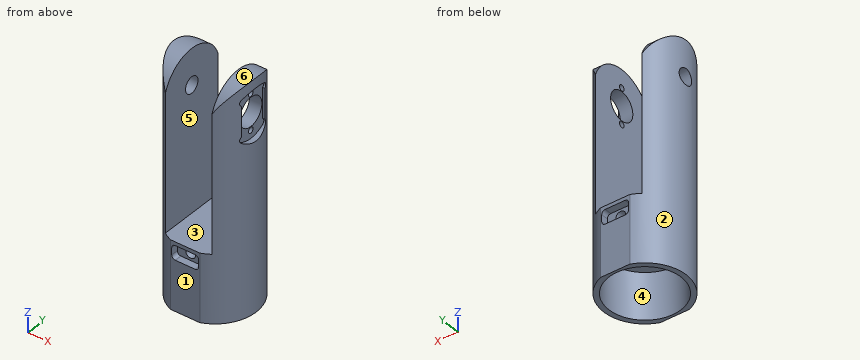
from build123d import *

# Parameters (mm, degrees)
F1_DEPTH  = 128
F3_W      = 26
F3_H      = 46
F4_DEPTH  = 90
F6_DEPTH  = 46.001
F8_DEPTH  = 3
F10_D     = 3.3
F10_DEPTH = 20
F10_TIP   = 0.9914200214
F11_R     = 8
F12_DEPTH = 25
F13_R     = 4.5
F14_DEPTH = 10.0010001
F15_R     = 20.15
F16_DEPTH = 26
F18_DEPTH = 4
F20_D     = 5.5
F20_DEPTH = 10
F20_TIP   = 1.6523667023
F22_DEPTH = 4
F24_D     = 5.5
F24_DEPTH = 10
F24_TIP   = 1.6523667023


with BuildPart() as f1:
    # F0 (on Top) → F1 (new body)
    with BuildSketch(Plane.XY):
        with BuildLine():
            Line((8.1700673192, 21.5), (-8.1700673192, 21.5))
            ThreePointArc((-8.1700673192, 21.5), (-23, 0), (-8.1700673192, -21.5))
            Line((-8.1700673192, -21.5), (8.1700673192, -21.5))
            ThreePointArc((8.1700673192, -21.5), (23, 0), (8.1700673192, 21.5))
        make_face()
    extrude(amount=F1_DEPTH)

    # F3 (on face) → F4 (cut)
    with BuildSketch(Plane.XY.offset(128)):
        Rectangle(F3_W, F3_H)
    extrude(amount=-F4_DEPTH, mode=Mode.SUBTRACT)

    # F5 (on offset) → F6 (cut, through all)
    with BuildSketch(Plane.YZ.offset(23)):
        with BuildLine():
            ThreePointArc((-19.9933908829, 108.5141215848), (-0.0190112138, 127.9999909643), (19.9923773451, 108.5521305014))
            Line((19.9923773451, 108.5521305014), (24.1833440959, 131.3719953258))
            Line((24.1833440959, 131.3719953258), (-19.9933908829, 131.3719953258))
            Line((-19.9933908829, 131.3719953258), (-19.9933908829, 108.5141215848))
        make_face()
    extrude(amount=-F6_DEPTH, mode=Mode.SUBTRACT)

    # F7 (on offset) → F8 (cut)
    with BuildSketch(Plane.YZ.offset(23)):
        with BuildLine():
            ThreePointArc((-8.55, 99.5196213389), (-9.3706896552, 97.9043111178), (-8.55, 96.2890008966))
            ThreePointArc((-8.55, 96.2890008966), (0, 93.5), (8.55, 96.2890008966))
            ThreePointArc((8.55, 96.2890008966), (9.3706896552, 97.9043111178), (8.55, 99.5196213389))
            Line((8.55, 99.5196213389), (8.55, 116.4803786611))
            ThreePointArc((8.55, 116.4803786611), (9.3706896552, 118.0956888822), (8.55, 119.7109991034))
            ThreePointArc((8.55, 119.7109991034), (0, 122.5), (-8.55, 119.7109991034))
            ThreePointArc((-8.55, 119.7109991034), (-9.3706896552, 118.0956888822), (-8.55, 116.4803786611))
            Line((-8.55, 116.4803786611), (-8.55, 99.5196213389))
        make_face()
    extrude(amount=-F8_DEPTH, mode=Mode.SUBTRACT)

    # F10
    with Locations(Plane.YZ.offset(20)):
        with Locations((0, 118), (0, 98)):
            Hole(F10_D / 2, depth=F10_DEPTH)
            with Locations((0, 0, -(F10_DEPTH + F10_TIP / 2))):  # 118° drill point
                Cone(0, F10_D / 2, F10_TIP, mode=Mode.SUBTRACT)

    # F11 (on face) → F12 (cut)
    with BuildSketch(Plane.YZ.offset(20)):
        with Locations((0, 108)):
            Circle(F11_R)
    extrude(amount=-F12_DEPTH, mode=Mode.SUBTRACT)

    # F13 (on face) → F14 (cut, through all)
    with BuildSketch(Plane.YZ.offset(-13)):
        with Locations((0, 108)):
            Circle(F13_R)
    extrude(amount=-F14_DEPTH, mode=Mode.SUBTRACT)

    # F15 (on face) → F16 (cut)
    with BuildSketch(Plane(origin=(0, 0, 0), x_dir=(1, 0, 0), z_dir=(0, 0, -1))):
        Circle(F15_R)
    extrude(amount=-F16_DEPTH, mode=Mode.SUBTRACT)

    # F17 (on face) → F18 (cut)
    with BuildSketch(Plane.XZ.offset(21.5)):
        with BuildLine():
            Line((5.5, 36), (-5.5, 36))
            ThreePointArc((-5.5, 36), (-6.9142135624, 35.4142135624), (-7.5, 34))
            Line((-7.5, 34), (-7.5, 30))
            ThreePointArc((-7.5, 30), (-6.9142135624, 28.5857864376), (-5.5, 28))
            Line((-5.5, 28), (5.5, 28))
            ThreePointArc((5.5, 28), (6.9142135624, 28.5857864376), (7.5, 30))
            Line((7.5, 30), (7.5, 34))
            ThreePointArc((7.5, 34), (6.9142135624, 35.4142135624), (5.5, 36))
        make_face()
    extrude(amount=-F18_DEPTH, mode=Mode.SUBTRACT)

    # F20
    with Locations(Plane.XZ.offset(17.5)):
        with Locations((0, 32)):
            Hole(F20_D / 2, depth=F20_DEPTH)
            with Locations((0, 0, -(F20_DEPTH + F20_TIP / 2))):  # 118° drill point
                Cone(0, F20_D / 2, F20_TIP, mode=Mode.SUBTRACT)

    # F21 (on face) → F22 (cut)
    with BuildSketch(Plane(origin=(0, 21.5, 0), x_dir=(-1, 0, 0), z_dir=(0, 1, 0))):
        with BuildLine():
            Line((5.5, 36), (-5.5, 36))
            ThreePointArc((-5.5, 36), (-6.9142135624, 35.4142135624), (-7.5, 34))
            Line((-7.5, 34), (-7.5, 30))
            ThreePointArc((-7.5, 30), (-6.9142135624, 28.5857864376), (-5.5, 28))
            Line((-5.5, 28), (5.5, 28))
            ThreePointArc((5.5, 28), (6.9142135624, 28.5857864376), (7.5, 30))
            Line((7.5, 30), (7.5, 34))
            ThreePointArc((7.5, 34), (6.9142135624, 35.4142135624), (5.5, 36))
        make_face()
    extrude(amount=-F22_DEPTH, mode=Mode.SUBTRACT)

    # F24
    with Locations(Plane(origin=(0, 17.5, 0), x_dir=(-1, 0, 0), z_dir=(0, 1, 0))):
        with Locations((0, 32)):
            Hole(F24_D / 2, depth=F24_DEPTH)
            with Locations((0, 0, -(F24_DEPTH + F24_TIP / 2))):  # 118° drill point
                Cone(0, F24_D / 2, F24_TIP, mode=Mode.SUBTRACT)


solid = f1.part
Input: part model. Units: mm. Frame: model coordinates. Face numbers are marked on the shaded views. A direction names the side the tool comes from. Give positions to 0.01 mm unless a question says otherwise; leave off trailing zeros. Order: outer loops, then holes, each group sorted by start corner. A loop starts at its lowest first (then second) coordinate and runs counter-clockwise, first axis right, second up. Notation, with made-up numbers: M -25,53 L 32,53 A35 ccw 32,87 Z; hole C -14,2.25 d7. An arc over 180 degrees is marked long. Answer as a JSON object with one key per item and string values.
1. Cut plane B-B, the plane z = 12.5. Output: boundary loops of the cut face in (x, y), and give its area (3 significant figures).
Result sheet:
{"outline": "M -8.17,-21.5 L 8.17,-21.5 A23 ccw 8.17,21.5 L -8.17,21.5 A23 ccw Z; hole C 0,0 d40.3", "area": "353 mm²"}
2. Cut plane A-A, the plane y = 0. State how many separate pieces and enclosed holes the cut face has, and give its area (4 significant figures).
Result sheet:
{"separate pieces": "5", "enclosed holes": "0", "area": "2,165 mm²"}
3. Cut plane C-C, the plane z = 108. Output: boundary loops of the cut face in (x, y), and give its area (3 significant figures).
Result sheet:
{"outline": "M -22.56,-4.5 A23 ccw -13,-18.97 L -13,-4.5 Z; M -22.56,4.5 L -13,4.5 L -13,18.97 A23 ccw Z; M 13,-18.97 A23 ccw 21.35,-8.55 L 20,-8.55 L 20,-8 L 13,-8 Z; M 13,8 L 20,8 L 20,8.55 L 21.35,8.55 A23 ccw 13,18.97 Z", "area": "290 mm²"}
4. Reachability of the marked faces 4, 5 and 6 from +Z, -Z, +X, -X, +Y, -Y: full face, straight path, thin tool, end or side. Return the list, or none.
Result sheet:
{"face 4": "-Z", "face 5": "+Z, +Y, -Y", "face 6": "+Z, +X, -X"}
5. First-contact query: P1, Ø2.5, axis at x = -1, z = 32, coming from the -Y side; P2, Ø2, axis at x = 2, y = -19, coming from the +Z side; P3, Ø1.1, axis at x = 21, z = 109.5, coming from the +Y side. Flat tips, straight axial feed; report the tip coordinate or a pass-through.
Result sheet:
{"P1": "y = -7.2", "P2": "z = 38", "P3": "y = 10.53"}
6. Cut plane D-D, the plane y = -13. Output: boundary loops of the cut face in (x, z), and give its area (3 significant figures).
Result sheet:
{"outline": "M -18.97,0 L -15.4,0 L -15.4,26 L 15.4,26 L 15.4,0 L 18.97,0 L 18.97,123.2 L 13,123.2 L 13,38 L -13,38 L -13,123.2 L -18.97,123.2 Z; hole C 0,32 d5.5", "area": "1,640 mm²"}
7. Pull-direction query (X, two-part tool) for the marked faces 1, 2 and 3; classes: +X half, -X half, draft (parallel to the pull), parting line (faces both ways), or undercut.
Result sheet:
{"face 1": "draft", "face 2": "-X half", "face 3": "undercut"}
8. Ray query, line 1 (Z direction, x = 17.25, y = 0); line 2 (Z direction, x = 0, y = 10); line 3 (Y direction, x = 0, z = 11). Return the intervals inside material, ascending. Write a range as [from, to].
Result sheet:
{"line 1": "[26, 96.35], [99.65, 100], [116, 116.35], [119.65, 128]", "line 2": "[26, 29.25], [34.75, 38]", "line 3": "[-21.5, -20.15], [20.15, 21.5]"}
